Input: part model. Units: mm. Frame: model coordinates. A direction names the side the tool comes from. Give positions to 0.01 mm unless a question says otherwise; leave off trailing zeros. Loops run counter-clockwise (first coordinate to the right, second up) from the corner with the lowest first, then second, coordinate; pieces in that order, holes last. Notation, with made-up numbers: (11, -13.75) -> (22, -13.75) arc R17 ccw to (22, 11.25) -> close; hole circle Ø10 at (-8.75, 83). An arc over 180 degrees is marked (long way). Answer as a JSON object with one key per item and string values. Group by question number.
```python
from build123d import *

# Parameters (mm, degrees)
SKETCH2_W           = 25.146
SKETCH2_H           = 17.78
BOSS_EXTRUDE1_DEPTH = 63.5
SKETCH3_W           = 20.574
SKETCH3_H           = 15.24
CUT_EXTRUDE1_DEPTH  = 59.69
SKETCH4_R           = 4.7625
BOSS_EXTRUDE2_DEPTH = 10.16
F_3DSKETCH1_R       = 5.08
CUT_EXTRUDE2_DEPTH  = 0.7366
SKETCH5_R           = 4.4577
SKETCH5_R_2         = 4.4704
BOSS_EXTRUDE3_DEPTH = 0.7366
SKETCH6_W           = 25.146
SKETCH6_H           = 23.368
CUT_EXTRUDE3_DEPTH  = 2.54


with BuildPart() as part:
    # Sketch2 → Boss-Extrude1 (new body)
    with BuildSketch(Plane(origin=(0, 0, 0), x_dir=(1, 0, 0), z_dir=(0, 1, 0))):
        Rectangle(SKETCH2_W, SKETCH2_H)
    extrude(amount=BOSS_EXTRUDE1_DEPTH)

    # Sketch3 → Cut-Extrude1 (cut)
    with BuildSketch(Plane(origin=(0, 63.5, 0), x_dir=(1, 0, 0), z_dir=(0, 1, 0))):
        with Locations((0, -1.27)):
            Rectangle(SKETCH3_W, SKETCH3_H)
    extrude(amount=-CUT_EXTRUDE1_DEPTH, mode=Mode.SUBTRACT)

    # Sketch4 → Boss-Extrude2 (add)
    with BuildSketch(Plane(origin=(0, 0, 0), x_dir=(-1, 0, 0), z_dir=(0, -1, 0))):
        with Locations(Location((6.223, 0, 0), (0, 0, 270))):
            Circle(SKETCH4_R)
        with Locations(Location((-6.223, 0, 0), (0, 0, 270))):
            Circle(SKETCH4_R)
    extrude(amount=BOSS_EXTRUDE2_DEPTH)

    # 3DSketch1 → Cut-Extrude2 (cut)
    with BuildSketch(Plane(origin=(-6.223, -6.35, 0), x_dir=(1, 0, 0), z_dir=(0, -1, 0))):
        Circle(F_3DSKETCH1_R)
        with Locations((12.446, 0)):
            Circle(F_3DSKETCH1_R)
    extrude(amount=CUT_EXTRUDE2_DEPTH, mode=Mode.SUBTRACT)


with BuildPart() as cut_extrude2_piece_1:
    # of the separate pieces the step leaves, piece 1, a body of its own (cut_extrude2_pieces)
    add(part.part.solids().sort_by_distance((-12.573, 0, -8.89))[0])



with BuildPart() as cut_extrude2_piece_2:
    # of the separate pieces the step leaves, piece 2, a body of its own (cut_extrude2_pieces)
    add(part.part.solids().sort_by_distance((6.223, -7.0866, 4.7625))[0])


with BuildPart() as cut_extrude2_piece_3:
    # of the separate pieces the step leaves, piece 3, a body of its own (cut_extrude2_pieces)
    add(part.part.solids().sort_by_distance((-6.223, -7.0866, 4.7625))[0])


with BuildPart() as cut_extrude2_piece_1_1:
    add(cut_extrude2_piece_1.part)

    add(cut_extrude2_piece_2.part)  # Boss-Extrude3 merges Cut-Extrude2 piece 2

    add(cut_extrude2_piece_3.part)  # Boss-Extrude3 merges Cut-Extrude2 piece 3
    # Sketch5 → Boss-Extrude3 (add)
    with BuildSketch(Plane(origin=(0, -6.35, 0), x_dir=(-1, 0, 0), z_dir=(0, -1, 0))):
        with Locations(Location((6.223, 0, 0), (0, 0, 90))):
            Circle(SKETCH5_R)
        with Locations(Location((-6.223, 0, 0), (0, 0, 90))):
            Circle(SKETCH5_R_2)
    extrude(amount=BOSS_EXTRUDE3_DEPTH)

    # Sketch6 → Cut-Extrude3 (cut)
    with BuildSketch(Plane(origin=(0, 0, -8.89), x_dir=(-1, 0, 0), z_dir=(0, 0, -1))):
        with Locations((0, 37.084)):
            Rectangle(SKETCH6_W, SKETCH6_H)
    extrude(amount=-CUT_EXTRUDE3_DEPTH, mode=Mode.SUBTRACT)


solid = cut_extrude2_piece_1_1.part
```
Q1. Section B-B on x = -3.75. Return the cut outline in (y, z).
Q2. Pull-direction query (Y, two-part tool) for faces 1 (the face through (-11, 22, 8.89)), 2 (the face through (6, -10.16, 0)), 3 (the face through (-10.575, -6.713, 0.966)), 4 (the face through (3.503, -6.713, 3.548)); classes: +Y half, -Y half, draft (parallel to the pull), parting line (faces both ways), or undercut.
Q3. Set-up query: faces 5 (the face through (0, 0, 0)), 6 (the face through (0, 56, -8.89)), 7 (the face through (0, 48.768, -8)), 8 (the face through (0, 3.81, 1)). Return all of +Z, -Z, +X, -X, +Y, -Y with unobstructed straight access to the full face (end or side cutting, diameter ignored); none if empty.
Q4. Section D-D on y = 50. Return the cut outline in (x, z).
Q5. Pin query (flat end, axial travel): pin 1 Ø3 at (x, z) = (4.5, 1) entering from +Y; pin 2 Ø3 at (x, z) = (5.5, -7.5) entering from -Y; pin 3 Ø7.5 at (x, y) = (-1.5, 53) entering from +Z; pin 4 Ø2 at (x, y) = (7, 46) entering from -Z. Return the tip coordinate at first contact, or that it passes through.
Q6. Section A-A on z = -7.25. Return the cut outline in (x, y).
Q7. Ray query, probe 1 along Y at (x, z) = (-7.5, -7.5); probe 2 along X at (y, z) = (29, -2.5); probe 3 along Y at (x, z) = (-2, 3.75). Return the intervals inside material, ascending.
Numbers:
{
 "1": {"outline": "(-10.16, -4.07) -> (-7.09, -4.07) -> (-7.09, -3.71) -> (-6.35, -3.71) -> (-6.35, -4.07) -> (0, -4.07) -> (0, -8.89) -> (25.4, -8.89) -> (25.4, -6.35) -> (3.81, -6.35) -> (3.81, 8.89) -> (0, 8.89) -> (0, 4.07) -> (-6.35, 4.07) -> (-6.35, 3.71) -> (-7.09, 3.71) -> (-7.09, 4.07) -> (-10.16, 4.07) -> close; (48.77, -8.89) -> (63.5, -8.89) -> (63.5, -6.35) -> (48.77, -6.35) -> close"},
 "2": {"face 1": "draft", "face 2": "-Y half", "face 3": "undercut", "face 4": "undercut"},
 "3": {"face 5": "-Y", "face 6": "-Z, +X, -X, +Y, -Y", "face 7": "-Z, +X, -X", "face 8": "+Z, +Y"},
 "4": {"outline": "(-12.57, -8.89) -> (12.57, -8.89) -> (12.57, 8.89) -> (10.29, 8.89) -> (10.29, -6.35) -> (-10.29, -6.35) -> (-10.29, 8.89) -> (-12.57, 8.89) -> close"},
 "5": {"pin 1": "stops at y = 3.81", "pin 2": "stops at y = 0", "pin 3": "stops at z = -6.35", "pin 4": "passes through"},
 "6": {"outline": "(-12.57, 0) -> (12.57, 0) -> (12.57, 25.4) -> (-12.57, 25.4) -> close; (-12.57, 48.77) -> (12.57, 48.77) -> (12.57, 63.5) -> (-12.57, 63.5) -> close"},
 "7": {"probe 1": "y = 0 to 25.4, 48.77 to 63.5", "probe 2": "x = -12.57 to -10.29, 10.29 to 12.57", "probe 3": "y = 0 to 3.81"}
}
